```python
from build123d import *

# Parameters (mm, degrees)
ESQUISSE1_R        = 7.125
ESQUISSE1_R_2      = 5.125
BOSS_EXTRU_1_DEPTH = 6
ESQUISSE1_3_R      = 1.75
BOSS_EXTRU_2_DEPTH = 2.5
CONG_1_R           = 3.5
CONG_2_R           = 10


with BuildPart() as part:
    # Esquisse1 → Boss.-Extru.1 (new body)
    with BuildSketch(Plane.XY):
        Circle(ESQUISSE1_R)
        Circle(ESQUISSE1_R_2, mode=Mode.SUBTRACT)
    extrude(amount=BOSS_EXTRU_1_DEPTH)

    # Esquisse1<3> → Boss.-Extru.2 (add)
    # profile 1 of 2: a face of its own
    with BuildSketch(Plane.XY):
        with BuildLine():
            Line((-15.998397436, 18.375), (-7.125, 0))
            ThreePointArc((-7.125, 0), (-5.038135816, 5.038135816), (0, 7.125))
            Line((0, 7.125), (0, 18.375))
            Line((0, 18.375), (-15.998397436, 18.375))
        make_face()
        with Locations((-10.4375, 14.625)):
            Circle(ESQUISSE1_3_R, mode=Mode.SUBTRACT)
    # profile 2 of 2: a face of its own
    with BuildSketch(Plane.XY):
        with BuildLine():
            ThreePointArc((0, 7.125), (5.038135816, 5.038135816), (7.125, 0))
            Line((7.125, 0), (15.998397436, 18.375))
            Line((15.998397436, 18.375), (0, 18.375))
            Line((0, 18.375), (0, 7.125))
        make_face()
        with Locations((10.4375, 14.625)):
            Circle(ESQUISSE1_3_R, mode=Mode.SUBTRACT)
    extrude(amount=BOSS_EXTRU_2_DEPTH)

    # Congé1
    cong_1_edges = [part.edges().sort_by_distance(p)[0] for p in [
        (15.998397436, 18.375, 1.25),
        (-15.998397436, 18.375, 1.25),
    ]]
    fillet(cong_1_edges, radius=CONG_1_R)

    # Congé2
    # the kernel refuses this fillet: 10 mm, written as the material it adds along each edge
    with BuildSketch(Plane(origin=(-7.125, 0, 0), x_dir=(0.08048003783871222, -0.9967562207026748, 0), z_dir=(0, 0, 1))) as cong_2_piece_1:
        with BuildLine():
            CenterArc((1.951640918, -9.967562207), CONG_2_R, 94.61615885, 16.543856934)
            Line((-1.658097624, -0.641802846), (0, 0))
            ThreePointArc((0, 0), (0.57342027, -0.023111927), (1.146840539, 0))
        make_face()
    extrude(amount=2.5)
    with BuildSketch(Plane(origin=(7.125, 0, 0), x_dir=(0.4348566812294863, 0.900499676174332, 0), z_dir=(0, 0, 1))) as cong_2_piece_2:
        with BuildLine():
            CenterArc((1.77797599, -10), CONG_2_R, 90, 16.543856934)
            ThreePointArc((-1.069515889, -0.413979449), (-0.526415143, -0.228543352), (0, 0))
            Line((0, 0), (1.77797599, 0))
        make_face()
    extrude(amount=2.5)


solid = part.part
```
Build history of the part. All positions in model axes, mm. A direction names the side the tool comes from. Round coordinates to 2 decimals unless told otherwise and drop trailing zeros. Order: outer loops, then holes, each group sorted by start corner. A loop starts at its lowest first (then second) coordinate and runs counter-clockwise, first axis right, second up. Notation, with made-up numbers: (-8, -30.75) - (8, -30.75) arc R28 cw to (8, -7.75) - close; hole circle Ø6 at (65.25, 79.5). An arc over 180 degrees is marked (long way). Use a Markdown table: item, result.
1) Pull direction X, two halves, no side cores. Call faces 3 (the face through (13.412, 16.693, 1.268)), 4 (the face through (-10.775, 7.559, 1.232)), 5 (the face through (-10.67, 16.36, 1.23)): pulls with the +X half, pulls with the -X half, needs draft (parallel to the pull), parting line crosses it, or undercut.
Recorded:
| item | result |
|---|---|
| face 3 | pulls with the +X half |
| face 4 | pulls with the -X half |
| face 5 | undercut |
2) Saw through at D-D on x = -3. Write the cut outline in (y, z) (3 decimals), and give its area (3 significant figures).
Recorded:
| item | result |
|---|---|
| outline | (-6.463, 0) - (-4.155, 0) - (-4.155, 6) - (-6.463, 6) - close; (4.155, 0) - (18.375, 0) - (18.375, 2.5) - (6.463, 2.5) - (6.463, 6) - (4.155, 6) - close |
| area | 57.5 mm² |
3) Saw through at A-A on x = 0. Write the cut outline in (y, z) (3 decimals).
Recorded:
| item | result |
|---|---|
| outline | (-7.125, 0) - (-5.125, 0) - (-5.125, 6) - (-7.125, 6) - close; (5.125, 0) - (18.375, 0) - (18.375, 2.5) - (7.125, 2.5) - (7.125, 6) - (5.125, 6) - close |
4) Wall check: L1, parallel to X at y = 15, z = 1.4; L2, parallel to X at y = 16, z = 1.3; L3, parallel to Y at x = 0, z = 4.35 (3 decimals). Give the ranges that are in metal, low to high.
Recorded:
| item | result |
|---|---|
| L1 | x = -13.92 to -12.15, -8.73 to 8.73, 12.15 to 13.92 |
| L2 | x = -13.74 to -11.52, -9.35 to 9.35, 11.52 to 13.74 |
| L3 | y = -7.125 to -5.125, 5.125 to 7.125 |
5) Saw through at B-B on y = 0. Write the cut outline in (x, z) (3 decimals).
Recorded:
| item | result |
|---|---|
| outline | (-7.288, 0) - (-5.125, 0) - (-5.125, 6) - (-7.125, 6) - (-7.125, 2.5) - (-7.288, 2.5) - close; (5.125, 0) - (7.288, 0) - (7.288, 2.5) - (7.125, 2.5) - (7.125, 6) - (5.125, 6) - close |
6) Flat gauge pins, fed straight in: pin 1 Ø9 at (x, y) = (0, 0) entering from -Z (3 decimals); pin 2 Ø3 at (y, z) = (11.5, 2) entering from +X. Where does each tip first touch, or does it go through?
Recorded:
| item | result |
|---|---|
| pin 1 | passes through |
| pin 2 | stops at x = 13.4 |
7) Saw through at C-C on z = 4.05. Write the cut outline in (x, y) (3 decimals), and give its area (3 significant figures).
Recorded:
| item | result |
|---|---|
| outline | circle Ø14.25 at (0, 0); hole circle Ø10.25 at (0, 0) |
| area | 77.0 mm² |
8) Tool access for faces 1 (the face through (7.372, 0.28, 1.232)), 2 (the face through (3.29, -6.32, 3.62)): list every direction of +Z, -Z, +X, -X, +Y, -Y with a clear straight run to the whole face (end or side of a thin tool).
Recorded:
| item | result |
|---|---|
| face 1 | +Z, -Z, +X, -Y |
| face 2 | +Z |
